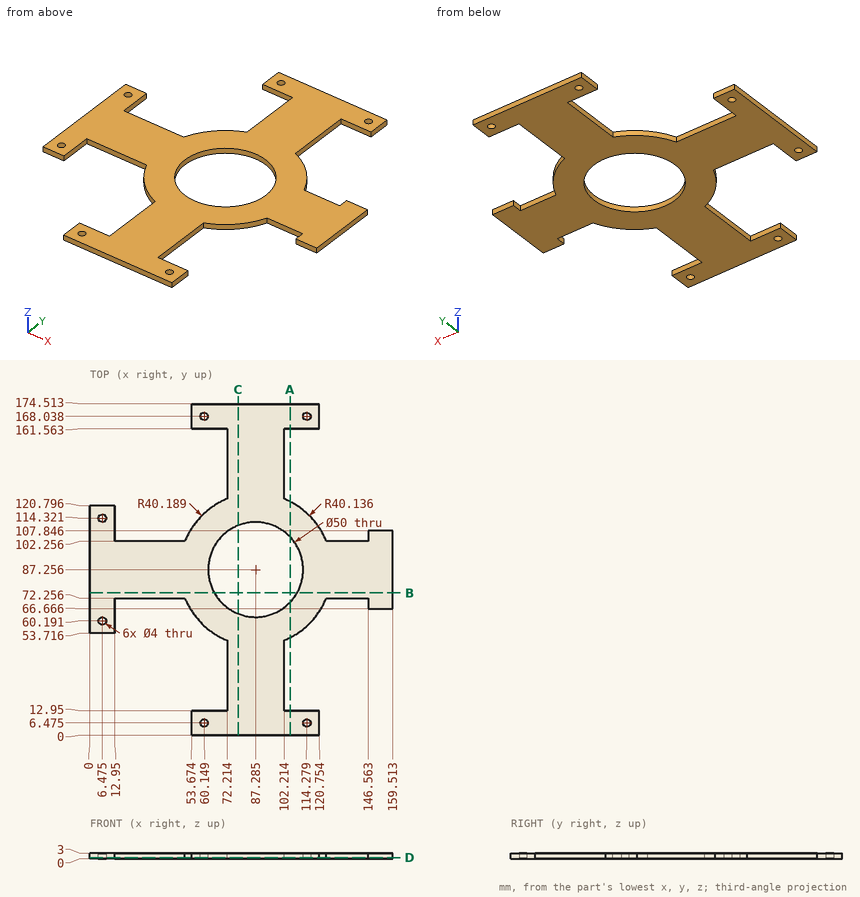
Geometry: see drawing. Coordinates: mm, zero at the bounding-box minimum. Give positions to 0.01 mm unless a question says otherwise; leave off trailing zeros. Order: outer loops, then holes, each group sorted by start corner. A loop starts at its lowest first (then second) coordinate and runs counter-clockwise, first axis right, second up. Notation, with made-up numbers: (0, 69) - (57, 69) arc R5 cw to (57, 77) - close; hole circle Ø4 at (-39.5, 60.5). An arc over 180 degrees is marked (long way). Write each question's results on one line, items separated by ' | '.
Item 1: Section B-B (y = 75). Return loops of the section in (x, z) (1 decimal), and give its area (3 significant figures).
A:
outline: (0, 0) - (65.5, 0) - (65.5, 3) - (0, 3) - close; (109.1, 0) - (159.5, 0) - (159.5, 3) - (109.1, 3) - close | area: 348 mm^2
Item 2: Material intervals for line 1 along X through (y, z) = (163, 0.65) (1 decimal); line 2 along Y through (x, z) = (43.5, 2.3); line 3 along X through (y, z) = (34.5, 1.15) (1 decimal), sorted ascending.
A:
line 1: x = 53.7 to 120.8 | line 2: y = 72.26 to 102.26 | line 3: x = 72.2 to 102.2
Item 3: Contact query for flat-ended pins moving along their axis: pin 1 Ø1 at (x, z) = (20.5, 1) entering from +Y; pin 2 Ø0.9 at (y, z) = (3.5, 1) entering from -X; pin 3 Ø0.9 at (y, z) = (65.5, 2) entering from +X; pin 4 Ø2.5 at (x, y) = (6.47, 114.32) entering from +Z. Output: stop coordinate, or through.
A:
pin 1: stops at y = 102.26 | pin 2: stops at x = 53.67 | pin 3: stops at x = 121.3 | pin 4: passes through
Item 4: Section D-D (z = 0.75). Give the number of separate pieces and of enclosed holes in the cut face, and give its area (3 significant figures).
A:
separate pieces: 1 | enclosed holes: 7 | area: 9,930 mm^2
Item 5: Section A-A (x = 105.5). Return loops of the section in (y, z).
A:
outline: (0, 0) - (12.95, 0) - (12.95, 3) - (0, 3) - close; (51.49, 0) - (70.13, 0) - (70.13, 3) - (51.49, 3) - close; (104.38, 0) - (123.02, 0) - (123.02, 3) - (104.38, 3) - close; (161.56, 0) - (174.51, 0) - (174.51, 3) - (161.56, 3) - close
Item 6: Section C-C (x = 78). Return loops of the section in (y, z) (1 decimal).
A:
outline: (0, 0) - (64, 0) - (64, 3) - (0, 3) - close; (110.5, 0) - (174.5, 0) - (174.5, 3) - (110.5, 3) - close
